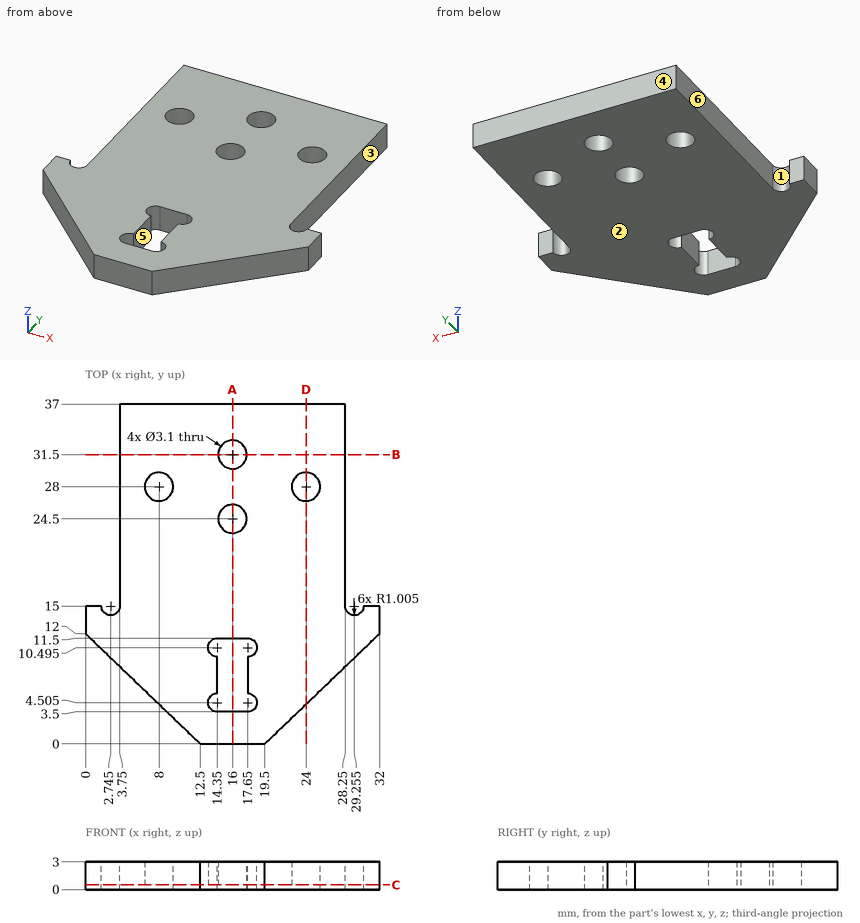
Geometry check sheet. Reference: drawing and pictorial views, mm from the part's lowest x, y, z. A direction names the side the tool comes from. Coordinates: 2 decimals unless noted, no trailing zeros. Write each loop counter-clockwise with the first axis right and the second up, starting at its lowest first coordinate (ties: lowest second). Pieces come first, ordered by that corner, then holes. Notation, with made-up numbers: (-38, -8) - (18, -8) arc R16 ccw to (18, 15) - close; hole circle Ø3 at (55.25, -16.75). An arc over 180 degrees is marked (long way). Write item = value, one per line.
Q1. Access from +Z, -Z, +X, -X, +Y, -Y to the whole of each face (thin tool, end or side, straight path). Record for the marked faces 4, 5 and 6.
Answer:
face_4 = +Z, -Z, +X, -X, +Y
face_5 = +Z, -Z
face_6 = +Z, -Z, -X, +Y
Q2. Material ranges on L1, parallel to Y at x = 16, z = 1.45; L2, parallel to Y at x = 13.5, z = 1.6; L3, parallel to X at y = 34.5, z = 2.4, recorded low to high. Write a range as from..to.
Answer:
L1 = 0..3.5, 11.5..22.95, 26.05..29.95, 33.05..37
L2 = 0..3.97, 5.04..9.96, 11.03..37
L3 = 3.75..28.25
Q3. Cross-section at D-D (x = 24). Enter the section's corners in (y, z).
Answer:
outline = (4.32, 0) - (26.45, 0) - (26.45, 3) - (4.32, 3) - close; (29.55, 0) - (37, 0) - (37, 3) - (29.55, 3) - close
Q4. Go/stop test with flat-tipped pins: pin 1 Ø1.9 at (x, y) = (24, 28) entering from +Z; pin 2 Ø1 at (y, z) = (23.5, 2) entering from +X; pin 3 Ø1.4 at (x, z) = (1, 2) entering from +Y; pin 4 Ø1 at (y, z) = (5, 1) entering from -X. Record where each tip stops, or that it passes through.
Answer:
pin_1 = through
pin_2 = 28.25
pin_3 = 15
pin_4 = 6.77
Q5. Cross-section at A-A (x = 16). Enter the section's corners in (y, z).
Answer:
outline = (0, 0) - (3.5, 0) - (3.5, 3) - (0, 3) - close; (11.5, 0) - (22.95, 0) - (22.95, 3) - (11.5, 3) - close; (26.05, 0) - (29.95, 0) - (29.95, 3) - (26.05, 3) - close; (33.05, 0) - (37, 0) - (37, 3) - (33.05, 3) - close
Q6. Cross-section at C-C (z = 0.5). Enter the section's corners in (x, y) (3 decimals), plus the area to 3 significant figures.
Answer:
outline = (0, 12) - (12.5, 0) - (19.5, 0) - (32, 12) - (32, 15) - (30.26, 15) arc R1.005 cw to (28.25, 15) - (28.25, 37) - (3.75, 37) - (3.75, 15) arc R1.005 cw to (1.74, 15) - (0, 15) - close; hole circle Ø3.1 at (8, 28); hole (14.35, 3.5) - (17.65, 3.5) arc R1.005 ccw to (17.65, 5.51) - (17.65, 9.49) arc R1.005 ccw to (17.65, 11.5) - (14.35, 11.5) arc R1.005 ccw to (14.35, 9.49) - (14.35, 5.51) arc R1.005 ccw to start; hole circle Ø3.1 at (16, 24.5); hole circle Ø3.1 at (16, 31.5); hole circle Ø3.1 at (24, 28)
area = 803 mm²
Q7. Mould release check, pull along X, two halves, no side actions. Record for the marked faces 1, 2 and 3: released by +X, released by -X, zero draft, split by the parting line, or undercut.
Answer:
face_1 = undercut
face_2 = zero draft
face_3 = released by +X
Q8. Cross-section at B-B (y = 31.5). Enter the section's corners in (x, z).
Answer:
outline = (3.75, 0) - (14.45, 0) - (14.45, 3) - (3.75, 3) - close; (17.55, 0) - (28.25, 0) - (28.25, 3) - (17.55, 3) - close
